The model under review builds one solid part; all positions refer to its coordinate system, in mm. A direction names the side the tool comes from. Round coordinates to 2 decimals unless told otherwise and drop trailing zeros. Order: outer loops, then holes, each group sorted by start corner. A loop starts at its lowest first (then second) coordinate and runs counter-clockwise, first axis right, second up.
1) Consider section D-D (z = 15.25). Give the boundary of the cut face in (x, y).
2) To check wall thickness, follow L1, parallel to X at y = 0.7, z = 15.25; L2, parallel to X at y = 0.9, z = 9.5; L3, parallel to X at y = 3.6, z = 16.5. State the ranges of each line that lie inside material, in increasing order.
3) Consider section A-A (y = 3.3). Give the boundary of the cut face in (x, z), then the cut area to 3 significant figures.
4) Machinability: for faces 1 (the face through (13.021, 2.669, 13.203)), 2 (the face through (16.63, 2.67, -12.7)), 3 (the face through (-13.269, 2.669, -17.455)), 4 (the face through (-16.63, 2.67, 12.7)), which of the approach directions +Z, -Z, +X, -X, +Y, -Y give a long, thin tool a straight path to every point of the face, cutting with its end or side? Answer none if there is none.
5) Mouldability with a two-part tool opening along X and no side actions: class faces 5 (the face through (-15.3, 2, 0)), 6 (the face through (0, 2, 18)), 7 (the face through (-13.295, 2.669, 17.47)) as pulls with the +X half, pulls with the -X half, needs draft (parallel to the pull), parting line crosses it, or undercut.
6) Clearance check with flat-ended pins moving along their axes: P1, Ø2.5, axis at x = -15.25, z = -15.25, coming from the -Y side; P2, Ø2, axis at y = 3, z = -15, coming from the -X side; P3, Ø3, axis at x = -16, z = 15, coming from the +Y side. State where each tip first meets the part, or that it passes through.
7) Consider section C-C (z = 0.5). Give the boundary of the cut face in (x, y).
8) Consider section B-B (y = 0.85). Give the boundary of the cut face in (x, z), then the cut area to 3 significant figures.
from build123d import *

# Parameters (mm, degrees)
SKETCH1_W           = 36
SKETCH1_H           = 36
BOSS_EXTRUDE1_DEPTH = 4
SKETCH2_R           = 1.5
CUT_EXTRUDE1_DEPTH  = 26.768197453
CUT_EXTRUDE3_DEPTH  = 2.7
CUT_EXTRUDE4_REACH  = 27.768
SKETCH4_W           = 2.6
SKETCH4_H           = 25.6


with BuildPart() as part:
    # Sketch1 → Boss-Extrude1 (new body)
    with BuildSketch(Plane(origin=(0, 0, 0), x_dir=(1, 0, 0), z_dir=(0, 1, 0))):
        Rectangle(SKETCH1_W, SKETCH1_H)
    extrude(amount=BOSS_EXTRUDE1_DEPTH)

    # Sketch2 → Cut-Extrude1 (cut, through all)
    with BuildSketch(Plane(origin=(0, 4, 0), x_dir=(1, 0, 0), z_dir=(0, 1, 0))):
        with Locations(Location((-15.25, 15.25, 0), (0, 0, 270))):
            Circle(SKETCH2_R)
        with Locations(Location((15.25, 15.25, 0), (0, 0, 270))):
            Circle(SKETCH2_R)
        with Locations(Location((15.25, -15.25, 0), (0, 0, 270))):
            Circle(SKETCH2_R)
        with Locations(Location((-15.25, -15.25, 0), (0, 0, 270))):
            Circle(SKETCH2_R)
    extrude(amount=-CUT_EXTRUDE1_DEPTH, mode=Mode.SUBTRACT)

    # Sketch3 → Cut-Extrude3 (cut)
    with BuildSketch(Plane(origin=(0, 4, 0), x_dir=(1, 0, 0), z_dir=(0, 1, 0))):
        Polygon((-15.25, 11.901368439), (-12.35, 13.575684219), (-12.35, 16.924315781), (-15.25, 18.598631561), (-18.15, 18.598631561), (-18.15, 16.924315781), (-18.15, 13.575684219), align=None)
        Polygon((15.26270162, 11.901392528), (18.156329948, 13.58669619), (18.143628328, 16.935303662), (18.143628328, 18.598607472), (15.23729838, 18.598607472), (12.343670052, 16.91330381), (12.356371672, 13.564696338), align=None)
        Polygon((18.17418246, -16.881713907), (18.125196925, -13.533440657), (15.201014465, -11.901726751), (12.32581754, -13.618286093), (12.374803075, -16.966559343), (15.298985535, -18.598273249), (18.17418246, -18.598273249), align=None)
        Polygon((-15.25, -18.598631561), (-12.35, -16.924315781), (-12.35, -13.575684219), (-15.25, -11.901368439), (-18.15, -13.575684219), (-18.15, -16.924315781), (-18.15, -18.598631561), align=None)
    extrude(amount=-CUT_EXTRUDE3_DEPTH, mode=Mode.SUBTRACT)

    # Sketch4 → Cut-Extrude4 (cut, up to next)
    with BuildSketch(Plane.XZ, mode=Mode.PRIVATE) as cut_extrude4_sk1:
        with Locations((-14, 0)):
            Rectangle(SKETCH4_W, SKETCH4_H)
    cut_extrude4_tool1 = extrude(cut_extrude4_sk1.sketch, amount=-CUT_EXTRUDE4_REACH, mode=Mode.PRIVATE) & part.part
    # Sketch4 → Cut-Extrude4 (cut, up to next)
    with BuildSketch(Plane.XZ, mode=Mode.PRIVATE) as cut_extrude4_sk2:
        with Locations((14, 0)):
            Rectangle(SKETCH4_W, SKETCH4_H)
    cut_extrude4_tool2 = extrude(cut_extrude4_sk2.sketch, amount=-CUT_EXTRUDE4_REACH, mode=Mode.PRIVATE) & part.part
    add(cut_extrude4_tool1.solids().sort_by_distance((-14, 0, 0))[0], mode=Mode.SUBTRACT)
    add(cut_extrude4_tool2.solids().sort_by_distance((14, 0, 0))[0], mode=Mode.SUBTRACT)


solid = part.part
Answer below:
1. outline: (-18, 0) - (-16.75, 0) - (-16.75, 1.3) - (-18, 1.3) - close; (-13.75, 0) - (13.75, 0) - (13.75, 1.3) - (12.35, 1.3) - (12.35, 4) - (-12.35, 4) - (-12.35, 1.3) - (-13.75, 1.3) - close; (16.75, 0) - (18, 0) - (18, 1.3) - (16.75, 1.3) - close
2. L1: x = -18 to -16.75, -13.75 to 13.75, 16.75 to 18
2. L2: x = -18 to -15.3, -12.7 to 12.7, 15.3 to 18
2. L3: x = -12.35 to 12.37
3. outline: (-18, -13.49) - (-15.3, -11.93) - (-15.3, 11.93) - (-18, 13.49) - close; (-14.21, -18) - (14.21, -18) - (12.34, -16.91) - (12.36, -13.56) - (13.69, -12.8) - (12.7, -12.8) - (12.7, 12.8) - (13.7, 12.8) - (12.33, 13.62) - (12.37, 16.97) - (14.23, 18) - (-14.21, 18) - (-12.35, 16.92) - (-12.35, 13.58) - (-13.69, 12.8) - (-12.7, 12.8) - (-12.7, -12.8) - (-13.69, -12.8) - (-12.35, -13.58) - (-12.35, -16.92) - close; (15.3, -11.92) - (18, -13.5) - (18, 13.46) - (15.3, 11.96) - close
3. area: 1,050 mm2
4. face 1: +Y
4. face 2: -Z, +Y
4. face 3: -X, +Y
4. face 4: +Z, +Y
5. face 5: undercut
5. face 6: needs draft
5. face 7: pulls with the -X half
6. P1: passes through
6. P2: stops at x = -12.35
6. P3: stops at y = 1.3
7. outline: (-18, 0) - (-15.3, 0) - (-15.3, 4) - (-18, 4) - close; (-12.7, 0) - (12.7, 0) - (12.7, 4) - (-12.7, 4) - close; (15.3, 0) - (18, 0) - (18, 4) - (15.3, 4) - close
8. outline: (-18, -18) - (18, -18) - (18, 18) - (-18, 18) - close; hole circle Ø3 at (-15.25, -15.25); hole circle Ø3 at (-15.25, 15.25); hole (-15.3, -12.8) - (-12.7, -12.8) - (-12.7, 12.8) - (-15.3, 12.8) - close; hole (12.7, -12.8) - (15.3, -12.8) - (15.3, 12.8) - (12.7, 12.8) - close; hole circle Ø3 at (15.25, -15.25); hole circle Ø3 at (15.25, 15.25)
8. area: 1,130 mm2
